Work out the finished part from the listing and answer in its coordinate system (mm). Round coordinates to 2 decimals unless told otherwise and drop trailing zeros. Write each loop counter-clockwise with the first axis right and the second up, starting at its lowest first coordinate (ties: lowest second). Pieces come first, ordered by that corner, then holes.
from build123d import *

# Parameters (mm, degrees)
SKETCH1_R           = 1.5
BOSS_EXTRUDE1_DEPTH = 1
SKETCH2_R           = 1.5
CUT_EXTRUDE1_DEPTH  = 10


with BuildPart() as part:
    # Sketch1 → Boss-Extrude1 (new body)
    with BuildSketch(Plane(origin=(0, 0, 0), x_dir=(1, 0, 0), z_dir=(0, 1, 0))):
        with BuildLine():
            Line((3, 0), (33, 0))
            ThreePointArc((33, 0), (35.121320344, 0.878679656), (36, 3))
            Line((36, 3), (36, 25))
            ThreePointArc((36, 25), (35.121320344, 27.121320344), (33, 28))
            Line((33, 28), (3, 28))
            ThreePointArc((3, 28), (0.878679656, 27.121320344), (0, 25))
            Line((0, 25), (0, 3))
            ThreePointArc((0, 3), (0.878679656, 0.878679656), (3, 0))
        make_face()
        with Locations((3, 25)):
            Circle(SKETCH1_R, mode=Mode.SUBTRACT)
        with Locations((3, 3)):
            Circle(SKETCH1_R, mode=Mode.SUBTRACT)
        with Locations((33, 25)):
            Circle(SKETCH1_R, mode=Mode.SUBTRACT)
        with Locations((33, 3)):
            Circle(SKETCH1_R, mode=Mode.SUBTRACT)
        with Locations((18, 22)):
            Circle(SKETCH1_R, mode=Mode.SUBTRACT)
        with Locations((18, 6)):
            Circle(SKETCH1_R, mode=Mode.SUBTRACT)
        with Locations((26, 14)):
            Circle(SKETCH1_R, mode=Mode.SUBTRACT)
        with Locations((10, 14)):
            Circle(SKETCH1_R, mode=Mode.SUBTRACT)
    extrude(amount=BOSS_EXTRUDE1_DEPTH)

    # Sketch2 → Cut-Extrude1 (cut)
    with BuildSketch(Plane(origin=(0, 1, 0), x_dir=(1, 0, 0), z_dir=(0, 1, 0))):
        with Locations((33, 14)):
            Circle(SKETCH2_R)
    extrude(amount=-CUT_EXTRUDE1_DEPTH, mode=Mode.SUBTRACT)


solid = part.part
Q1. Find section A-A (z = -22). Determine the outline of the cut face in (x, y), plus the area to 3 significant figures.
Q2. Find section C-C (x = 10). Determine the outline of the cut face in (y, z).
Q3. Find section B-B (y = 0.5). Count the separate pieces of the cut face and the enclosed holes in it, plus the area to 3 significant figures.
Q4. Find section D-D (x = 18). Determine the outline of the cut face in (y, z).
Q5. The mould has two halves that part along X. Classify faces 1 (the face through (18.2, 0.5, -28)), 2 (the face through (16.5, 0.49, -6.07)), 3 (the face through (0.86, 0.49, -0.9)): +X half, -X half, draft (parallel to the pull), parting line (faces both ways), or undercut.
Q6. Given pin 1 (2.5 mm diameter, centred on x = 33, z = -14, fed in from +Y), flat-ended and moving along its own axis, determine where the tip first touches the part or whether it passes through.
Q7. Find the intervals of material crossed by L1, parallel to Z at x = 33, y = 0.5; L2, parallel to X at y = 0.4, z = -14; L3, parallel to Z at x = 3, y = 0.5, in increasing order.
Report:
1. outline: (0, 0) - (16.5, 0) - (16.5, 1) - (0, 1) - close; (19.5, 0) - (36, 0) - (36, 1) - (19.5, 1) - close
1. area: 33.0 mm2
2. outline: (0, -28) - (1, -28) - (1, -15.5) - (0, -15.5) - close; (0, -12.5) - (1, -12.5) - (1, 0) - (0, 0) - close
3. separate pieces: 1
3. enclosed holes: 9
3. area: 937 mm2
4. outline: (0, -28) - (1, -28) - (1, -23.5) - (0, -23.5) - close; (0, -20.5) - (1, -20.5) - (1, -7.5) - (0, -7.5) - close; (0, -4.5) - (1, -4.5) - (1, 0) - (0, 0) - close
5. face 1: draft
5. face 2: undercut
5. face 3: -X half
6. pin 1: passes through
7. L1: z = -28 to -26.5, -23.5 to -15.5, -12.5 to -4.5, -1.5 to 0
7. L2: x = 0 to 8.5, 11.5 to 24.5, 27.5 to 31.5, 34.5 to 36
7. L3: z = -28 to -26.5, -23.5 to -4.5, -1.5 to 0
